Read the model definition and answer for the solid it produces. Units are mm, in the model's axes. Face numbers are marked on the shaded views. A direction names the side the tool comes from. Coordinates: 2 decimals unless noted, no trailing zeros. Loops run counter-clockwise (first coordinate to the right, second up) from the corner with the lowest first, then second, coordinate; pieces in that order, holes last. Notation, with made-up numbers: (73, 74.25) -> (85, 74.25) arc R26 ccw to (85, 107.25) -> close; hole circle Ø2 at (76.5, 42). An arc over 180 degrees is marked (long way). Answer as a JSON object with one key per item and string values. Group by question number.
Q1. For the marked faces 1, 2 and 3, determine the directions among +Z, -Z, +X, -X, +Y, -Y from which every point of the face is accessible in a straight line to the end or side of a thin tool.
Q2. Each of these flat-tipped pins is pushed along its axis until it touches: P1, Ø5.5, axis at x = 0, z = 21, coming from the +Y side; P2, Ø8, axis at y = -28.5, z = -10.5, coming from the +X side; P3, Ø4, axis at x = -23.5, y = -13, coming from the -Z side; P4, Ø12, axis at y = 27, z = 14.5, coming from the +X side. Where does it stop, or does it pass through?
Q3. Straight lines are drawn through the part: line 1 along Y through (x, z) = (0, 8); line 2 along X through (y, z) = (-14.5, -2); line 3 along Y through (x, z) = (0, 13). For each, find the intervals that lie inside material, in ascending order. Write a range as [from, to].
Q4. Determine the mould class of the marked faces 4, 5, 6 and 7 for opening direction Z: released by +Z, released by -Z, zero draft, split by the parting line, or undercut.
Q5. The part is cut by section D-D on z = -9. Write down the section's boundary in (x, y).
Q6. The part is cut by section A-A on x = 0. State how many separate pieces and enclosed holes the cut face has, and give its area (3 significant figures).
Q7. The part is cut by section C-C on z = 21. Write down the section's boundary in (x, y), and give its area (3 significant figures).
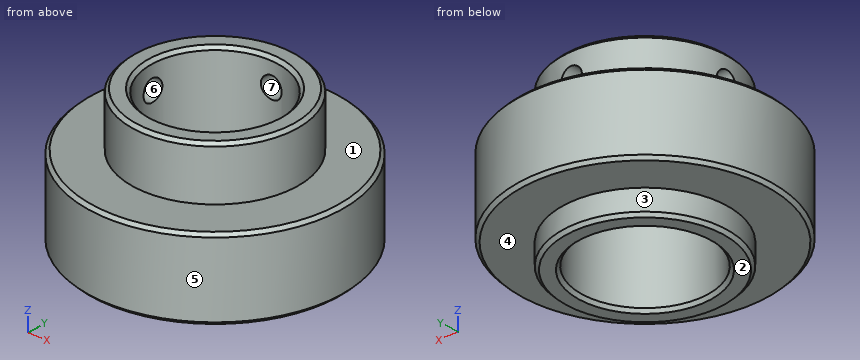
from build123d import *

# Parameters (mm, degrees)
F0_R          = 26
F0_R_2        = 20
F1_DEPTH      = 29.2
F1_DEPTH_BACK = 20
F2_SIZE       = 1
F4_D          = 6.6
F4_DEPTH      = 26.001
F6_D          = 6.6
F6_DEPTH      = 26.0010001
F7_R          = 40
F8_DEPTH      = 12.5
F8_DEPTH_BACK = 12.5
F9_DEPTH      = 25
F10_SIZE      = 1


with BuildPart() as f1:
    # F0 (on Top) → F1 (new body, two sides)
    with BuildSketch(Plane.XY) as f1_sk:
        Circle(F0_R)
        Circle(F0_R_2, mode=Mode.SUBTRACT)
    extrude(amount=F1_DEPTH)
    extrude(f1_sk.sketch, amount=-F1_DEPTH_BACK)

    # F2
    f2_edges = [f1.edges().sort_by_distance(p)[0] for p in [
        (-20, 0, 29.2),
        (-26, 0, 29.2),
        (-20, 0, -20),
        (-26, 0, -20),
    ]]
    chamfer(f2_edges, length=F2_SIZE)

    # F4 (through all, one way)
    with BuildSketch(Plane.XZ):
        with Locations((0, 21)):
            Circle(F4_D / 2)
    extrude(amount=-F4_DEPTH, mode=Mode.SUBTRACT)

    # F6 (through all, one way)
    with BuildSketch(Plane.YZ):
        with Locations((0, 21)):
            Circle(F6_D / 2)
    extrude(amount=-F6_DEPTH, mode=Mode.SUBTRACT)

    # F7 (on Top) → F8 (join, two sides)
    with BuildSketch(Plane.XY) as f8_sk:
        Circle(F7_R)
    extrude(amount=F8_DEPTH)
    extrude(f8_sk.sketch, amount=-F8_DEPTH_BACK)

    # F9 (cut): a face of the model
    f9_faces = [f1.faces().sort_by_distance(p)[0] for p in [
        (0, 0, 12.5),
    ]]
    extrude(f9_faces, amount=-F9_DEPTH, mode=Mode.SUBTRACT)

    # F10
    f10_edges = [f1.edges().sort_by_distance(p)[0] for p in [
        (-40, 0, 12.5),
        (-40, 0, -12.5),
    ]]
    chamfer(f10_edges, length=F10_SIZE)


solid = f1.part
Final values:
{
 "1": {"face 1": "+Z", "face 2": "-Z, +X, -X, +Y, -Y", "face 3": "-Z"},
 "2": {"P1": "stops at y = -19.81", "P2": "stops at x = 31.62", "P3": "stops at z = -20", "P4": "stops at x = 33.53"},
 "3": {"line 1": "y = [-40, -20], [20, 40]", "line 2": "x = [-37.28, -13.77], [13.77, 37.28]", "line 3": "y = [-26, -20], [20, 26]"},
 "4": {"face 4": "released by -Z", "face 5": "zero draft", "face 6": "undercut", "face 7": "undercut"},
 "5": {"outline": "circle Ø80 at (0, 0); hole circle Ø40 at (0, 0)"},
 "6": {"separate pieces": "3", "enclosed holes": "0", "area": "1,240 mm2"},
 "7": {"outline": "(-25.79, -3.3) arc R26 ccw (long way) to (3.3, 25.79) -> (3.3, 19.73) arc R20 cw (long way) to (-19.73, -3.3) -> close; (-25.79, 3.3) -> (-19.73, 3.3) arc R20 cw to (-3.3, 19.73) -> (-3.3, 25.79) arc R26 ccw to start", "area": "788 mm2"}
}
